Can you work these out from the model? Positions are in its coordinate system, mm. Face numbers are marked on the shaded views. A direction names the side the tool comes from. Give positions to 0.01 mm unless a question says otherwise; leave off trailing zeros. Write each loop counter-clockwise with the first axis right and the second up, starting at its lowest first coordinate (ties: lowest second). Pieces come first, ordered by that corner, then holes. Notation, with made-up numbers: M 22.25,39.25 L 79.25,39.25 A12 cw 79.25,58.25 Z; hole C 6.25,-36.75 d9. An arc over 180 degrees is marked long. Write each question's results on one line, items separated by ' | '.
Autodesk Inventor part; units mm, degrees
ref_plane "SCHRAUBE_XY" through (0, 0, 0) normal (-1, 0, 0) x (0, 0, -1)
ref_plane "SCHRAUBE_YZ" through (0, 0, 0) normal (0, 0, -1) x (0, -1, 0)
ref_plane "SCHRAUBE_ZX" through (0, 0, 0) normal (0, -1, 0) x (-1, 0, 0)
sketch "Sketch_1" plane through (0, 0, 0) normal (0, 0, 1) x (1, 0, 0)
  line L0 (30, 0) -> (-10, 0)
  line L1 (-10, 0) -> (-10, 7.5)
  arc A0 (-9.5, 8) -> (-10, 7.5) centre (-9.5, 7.5) ccw
  line L2 (-9.5, 8) -> (0, 8)
  line L3 (0, 8) -> (0, 5)
  line L4 (0, 5) -> (29.08, 5)
  line L5 (29.08, 5) -> (30, 4.08)
  line L6 (30, 4.08) -> (30, 0)
  line L7 (30, 0) -> (-10, 0)
revolve "Revolution1" add sketch "Sketch_1" angle 360 about axis through (30, 0, 0) along (1, 0, 0)
thread "Thread1"
sketch "Sketch_3" plane through (-10, 0, 0) normal (-1, 0, 0) x (0, 1, 0)
  line L0 (-4, -2.3094) -> (0, -4.6188)
  line L1 (0, -4.6188) -> (4, -2.3094)
  line L2 (4, -2.3094) -> (4, 2.3094)
  line L3 (4, 2.3094) -> (0, 4.6188)
  line L4 (0, 4.6188) -> (-4, 2.3094)
  line L5 (-4, 2.3094) -> (-4, -2.3094)
extrude "Extrusion1" cut sketch "Sketch_3" against normal blind 4
sketch "Sketch_4" plane through (0, 0, 0) normal (0, 0, 1) x (1, 0, 0)
  line L0 (30, 0) -> (20, 0)
  line L1 (20, 8.5) -> (20, 5)
  line L2 (20, 5) -> (30, 5)
  line L3 (30, 5) -> (30, 6.4805)
  arc A0 (30, 6.4805) -> (29.7192, 6.9299) centre (29.5, 6.4805) ccw
  line L4 (29.7192, 6.9299) -> (26.5, 8.5)
  line L5 (26.5, 8.5) -> (25.9306, 10.625)
  line L6 (25.9306, 10.625) -> (20.5694, 10.625)
  line L7 (20.5694, 10.625) -> (20, 8.5)
revolve "Revolution2" add sketch "Sketch_4" angle 360 about axis through (30, 0, 0) along (1, 0, 0)
sketch "Sketch_5" plane through (30, 0, 0) normal (1, 0, 0) x (0, 0, -1)
  line L0 (-17, -17) -> (17, -17)
  line L1 (17, -17) -> (17, 17)
  line L2 (17, 17) -> (-17, 17)
  line L3 (-17, 17) -> (-17, -17)
  line L4 (-8.5, -4.9075) -> (0, -9.815)
  line L5 (0, -9.815) -> (8.5, -4.9075)
  line L6 (8.5, -4.9075) -> (8.5, 4.9075)
  line L7 (8.5, 4.9075) -> (0, 9.815)
  line L8 (0, 9.815) -> (-8.5, 4.9075)
  line L9 (-8.5, 4.9075) -> (-8.5, -4.9075)
extrude "Extrusion2" cut sketch "Sketch_5" against normal blind 10
ref_plane "SCHRAUBE_XY" through (0, 0, 0) normal (-1, 0, 0) x (0, 0, -1)
ref_plane "SCHRAUBE_YZ" through (0, 0, 0) normal (0, 0, -1) x (0, -1, 0)
ref_plane "SCHRAUBE_ZX" through (0, 0, 0) normal (0, -1, 0) x (-1, 0, 0)
properties part number "M10x30"
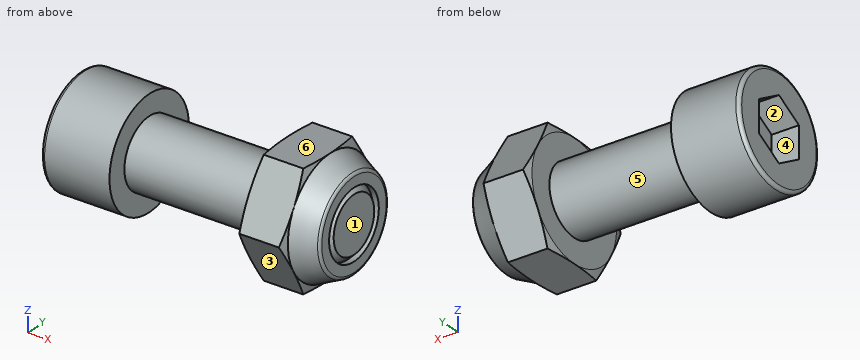
Item 1: I want a section at A-A, the plane x = 25. Please give me the cut outline in (y, z) (1 decimal), and give its area (3 significant figures).
Geometry says:
outline: M -9.8,0 L -4.9,-8.5 L 4.9,-8.5 L 9.8,0 L 4.9,8.5 L -4.9,8.5 Z | area: 250 mm2
Item 2: For the marked faces 4, 5 and 6, which set-ups out of +Z, -Z, +X, -X, +Y, -Y let a thin tool reach every point of the face, with its end or its side?
Geometry says:
face 4: -X | face 5: none | face 6: +Z, +X, -X, +Y, -Y
Item 3: Thinking about a two-plate mould opening in Y: for the marked faces 1, 2 and 3, which applies, +Y half, -Y half, draft (parallel to the pull), parting line (faces both ways), or undercut?
Geometry says:
face 1: draft | face 2: undercut | face 3: -Y half
Item 4: If I drill on line 1 (X direction, y = 4.5, z = -3.25); line 2 (Z direction, x = 29.35, y = 0); line 3 (Y direction, x = -7, z = -0.25), over which ranges is the centre line in solid material (lowest first)? Write a range as from..to.
Geometry says:
line 1: x = -10..0, 20..30 | line 2: z = -7.11..-5, -4.73..4.73, 5..7.11 | line 3: y = -8..-4, 4..8
Item 5: I'm going to push flat-ended pins straight in: pin 1 (4 mm diameter, centred on x = 11, y = 2, fed in from +Z); pin 2 (4.5 mm diameter, centred on x = -8.5, z = 0.5, fed in from +Y); pin 3 (6 mm diameter, centred on x = 22.5, z = -5, fed in from +Y). Where does each tip first touch, or does it pass through?
Geometry says:
pin 1: stops at z = 5 | pin 2: stops at y = 8 | pin 3: stops at y = 8.66
